Model file for the job. Use its own axes, mm. A direction names the side the tool comes from. Coordinates: 2 decimals unless noted, no trailing zeros. Order: outer loops, then holes, each group sorted by start corner. A loop starts at its lowest first (then second) coordinate and runs counter-clockwise, first axis right, second up. Notation, with made-up numbers: (79, 26) -> (130, 26) arc R8 ccw to (130, 31) -> close; hole circle Ø9 at (-29, 38). An arc over 180 degrees is marked (long way). Return JSON: item names as keys, results as strings. Group by question number.
1) Flat gauge pins, fed straight in: pin 1 (5 mm diameter, centred on y = -8, z = -9.5, fed in from -X); pin 2 (5.5 mm diameter, centred on x = -25, z = 0, fed in from +Y); pin 3 (8.5 mm diameter, centred on x = -10, z = 15, fed in from -Y). Where does each tip first touch, or does it go through?
2) Which spindle directions (+Z, -Z, +X, -X, +Y, -Y) get a long thin tool onto all of the face, cutting with end or side? Do faces 1 (the cylindrical face through (-6.583, -7.888, -0.759)), 2 (the flat face through (-7.8, 1, 15)), 3 (the cylindrical face through (-19.293, 1.014, 9.091)). Say none if no direction does.
3) Pull direction Z, two halves, no side cores. Call faces 4 (the flat face through (-5, 2, 0)), 5 (the flat face through (6, -7, -20)), 6 (the cylindrical face through (-25.15, 1.51, -3.17)): +Z half, -Z half, draft (parallel to the pull), parting line (faces both ways), or undercut.
4) Cut at C-C (z = -15). Write the cut outline in (x, y), and give its area (3 significant figures).
5) Cut at B-B (y = -14.25). Write the cut outline in (x, z).
6) Probe line 1 (Z direction, x = 10, y = -11.75); line 2 (X direction, y = -9, z = -15); line 3 (Z direction, x = -10, y = 1.35) (3 decimals). List the from-to ranges inside material, lowest first.
7) Cut at A-A (x = -25). Write the cut outline in (y, z) (3 decimals).
8) Cut at D-D (x = 10). Write the cut outline in (y, z).
from build123d import *

# Parameters (mm, degrees)
SKETCH1_W             = 60
SKETCH1_H             = 40
BOSS_EXTRUDE1_DEPTH   = 2
CUT_EXTRUDE1_DEPTH    = 14
SKETCH5_R             = 3.5
BOSS_EXTRUDE3_DEPTH   = 16
SKETCH6_W             = 30
SKETCH6_H             = 40
BOSS_EXTRUDE4_DEPTH   = 16
SKETCH8_R             = 3.175
CUT_EXTRUDE2_DEPTH    = 1
SKETCH9_W             = 10
SKETCH9_H             = 40
CUT_EXTRUDE3_DEPTH    = 20
F_3_0MM_DOWEL_HOLE1_D = 3


with BuildPart() as part:
    # Sketch1 → Boss-Extrude1 (new body)
    with BuildSketch(Plane(origin=(0, 0, 0), x_dir=(1, 0, 0), z_dir=(0, 1, 0))):
        Rectangle(SKETCH1_W, SKETCH1_H)
    extrude(amount=BOSS_EXTRUDE1_DEPTH)

    # Sketch4 → Cut-Extrude1 (cut)
    with BuildSketch(Plane(origin=(0, 2, 0), x_dir=(1, 0, 0), z_dir=(0, 1, 0))):
        with BuildLine():
            ThreePointArc((-23, 0), (-19.192388155, -9.192388155), (-10, -13))
            ThreePointArc((-10, -13), (-8, -15), (-10, -17))
            ThreePointArc((-10, -17), (-22.02081528, -12.02081528), (-27, 0))
            ThreePointArc((-27, 0), (-25, 2), (-23, 0))
        make_face()
    extrude(amount=-CUT_EXTRUDE1_DEPTH, mode=Mode.SUBTRACT)

    # Sketch5 → Boss-Extrude3 (add)
    with BuildSketch(Plane.XZ):
        with Locations(Location((-10, 0, 0), (0, 0, 90))):
            Circle(SKETCH5_R)
    extrude(amount=BOSS_EXTRUDE3_DEPTH)

    # Sketch6 → Boss-Extrude4 (add)
    with BuildSketch(Plane.XZ):
        with Locations((15, 0)):
            Rectangle(SKETCH6_W, SKETCH6_H)
    extrude(amount=BOSS_EXTRUDE4_DEPTH)

    # Sketch8 → Cut-Extrude2 (cut)
    with BuildSketch(Plane(origin=(0, 2, 0), x_dir=(1, 0, 0), z_dir=(0, 1, 0))):
        with Locations((-25, 0)):
            Circle(SKETCH8_R)
        with Locations((-10, -15)):
            Circle(SKETCH8_R)
    extrude(amount=-CUT_EXTRUDE2_DEPTH, mode=Mode.SUBTRACT)

    # Sketch9 → Cut-Extrude3 (cut)
    with BuildSketch(Plane(origin=(0, 2, 0), x_dir=(1, 0, 0), z_dir=(0, 1, 0))):
        with Locations((25, 0)):
            Rectangle(SKETCH9_W, SKETCH9_H)
    extrude(amount=-CUT_EXTRUDE3_DEPTH, mode=Mode.SUBTRACT)

    # Ø3.0mm Dowel Hole1 (through all)
    with Locations(Plane(origin=(0, 2, 0), x_dir=(1, 0, 0), z_dir=(0, 1, 0))):
        with Locations((10, 15), (10, -15)):
            Hole(F_3_0MM_DOWEL_HOLE1_D / 2)


solid = part.part
Answers below:
{
 "1": {"pin 1": "stops at x = 0", "pin 2": "stops at y = 1", "pin 3": "stops at y = 0"},
 "2": {"face 1": "-Y", "face 2": "+Y", "face 3": "+Y, -Y"},
 "3": {"face 4": "draft", "face 5": "-Z half", "face 6": "undercut"},
 "4": {"outline": "(-30, 0) -> (0, 0) -> (0, -16) -> (8.5, -16) -> (8.5, 2) -> (-30, 2) -> close; (11.5, -16) -> (20, -16) -> (20, 2) -> (11.5, 2) -> close", "area": "366 mm^2"},
 "5": {"outline": "circle Ø7 at (-10, 0); (0, -20) -> (20, -20) -> (20, 20) -> (0, 20) -> close; hole circle Ø3 at (10, -15); hole circle Ø3 at (10, 15)"},
 "6": {"line 1": "z = -20 to -16.5, -13.5 to 13.5, 16.5 to 20", "line 2": "x = 0 to 8.5, 11.5 to 20", "line 3": "z = -20 to 11.825, 18.175 to 20"},
 "7": {"outline": "(0, -20) -> (2, -20) -> (2, -3.175) -> (1, -3.175) -> (1, -2) -> (0, -2) -> close; (0, 8) -> (2, 8) -> (2, 20) -> (0, 20) -> close"},
 "8": {"outline": "(-16, -20) -> (2, -20) -> (2, -16.5) -> (-16, -16.5) -> close; (-16, -13.5) -> (2, -13.5) -> (2, 13.5) -> (-16, 13.5) -> close; (-16, 16.5) -> (2, 16.5) -> (2, 20) -> (-16, 20) -> close"}
}
